```python
from build123d import *

# Parameters (mm, degrees)
SKETCH_1_W          = 37
SKETCH_1_H          = 30
SKETCH_1_R          = 1.5
EXTRUDE_1_DEPTH     = 10
SKETCH_2_R          = 1.5
CUT_EXTRUDE_1_DEPTH = 6
SKETCH_3_W          = 30
SKETCH_3_H          = 8
CUT_EXTRUDE_2_DEPTH = 3
SKETCH_4_R          = 1
CUT_EXTRUDE_3_DEPTH = 7


with BuildPart() as part:
    # Эскиз1 → Бобышка-Вытянуть1 (new body)
    with BuildSketch(Plane(origin=(0, 0, 0), x_dir=(1, 0, 0), z_dir=(0, 1, 0))):
        with Locations((18.5, 15)):
            Rectangle(SKETCH_1_W, SKETCH_1_H)
        with Locations(Location((26.949747468, 19.949747468, 0), (0, 0, 270))):
            Circle(SKETCH_1_R, mode=Mode.SUBTRACT)
        with Locations(Location((17.050252532, 19.949747468, 0), (0, 0, 270))):
            Circle(SKETCH_1_R, mode=Mode.SUBTRACT)
        with Locations(Location((26.949747468, 10.050252532, 0), (0, 0, 270))):
            Circle(SKETCH_1_R, mode=Mode.SUBTRACT)
        with Locations(Location((17.050252532, 10.050252532, 0), (0, 0, 270))):
            Circle(SKETCH_1_R, mode=Mode.SUBTRACT)
    extrude(amount=EXTRUDE_1_DEPTH)

    # Эскиз2 → Вырез-Вытянуть1 (cut)
    with BuildSketch(Plane(origin=(37, 0, 0), x_dir=(0, 0, -1), z_dir=(1, 0, 0))):
        with Locations((8, 5)):
            Circle(SKETCH_2_R)
        with Locations((22, 5)):
            Circle(SKETCH_2_R)
    extrude(amount=-CUT_EXTRUDE_1_DEPTH, mode=Mode.SUBTRACT)

    # Эскиз3 → Вырез-Вытянуть2 (cut)
    with BuildSketch(Plane.ZY):
        with Locations((-15, 6)):
            Rectangle(SKETCH_3_W, SKETCH_3_H)
    extrude(amount=-CUT_EXTRUDE_2_DEPTH, mode=Mode.SUBTRACT)

    # Эскиз4 → Вырез-Вытянуть3 (cut)
    with BuildSketch(Plane.ZY):
        with Locations((-20, 5.4)):
            Circle(SKETCH_4_R)
        with Locations((-10, 5.4)):
            Circle(SKETCH_4_R)
    extrude(amount=-CUT_EXTRUDE_3_DEPTH, mode=Mode.SUBTRACT)


solid = part.part
```
Could you check a few things on this model? Use its own coordinates, in mm. A direction names the side the tool comes from. Give positions to 0.01 mm unless a question says otherwise; leave off trailing zeros. Order: outer loops, then holes, each group sorted by start corner. A loop starts at its lowest first (then second) coordinate and runs counter-clockwise, first axis right, second up.
Q1. Suppose I cut it at B-B, the plane y = 5. Write out the boundary of the cut face in (x, z), and give its area (3 significant figures).
Q2. For faces 4 (the cylindrical face through (4.972, 4.424, -10.217)), 5 (the flat face through (3, 6, -15)), 6 (the flat face through (31, 5, -8)), which set-ups out of +Z, -Z, +X, -X, +Y, -Y let a thin tool reach every point of the face, with its end or its side?
Q3. Suppose I cut it at D-D, the plane x = 16.5. Write out the boundary of the cut face in (y, z), and give its area (3 significant figures).
Q4. If I drill on line 1 along Z through (x, y) = (17, 8); line 2 along X through (y, z) = (0.75, -20.5); line 3 along Z through (x, y) = (18, 3), over which ranges is the centre line in solid material (lowest first)?
Q5. I'm going to push flat-ended pins straight in: P1, Ø1.5, axis at y = 4.5, z = -8.5, coming from the +X side; P2, Ø3.5, axis at x = 1, z = -14, coming from the +Y side; P3, Ø4, axis at y = 7.5, z = -21.5, coming from the -X side. Where does each tip first touch, or does it pass through?
Q6. We'd pull the mould along Y, two halves only. Please class faces 1 (the flat face through (31, 5, -22)), 2 (the flat face through (1, 2, -15)), 3 (the flat face through (18, 5, 0)): +Y half, -Y half, draft (parallel to the pull), parting line (faces both ways), or undercut.
Q7. Suppose I cut it at A-A, the plane x = 3.5. Write out the boundary of the cut face in (y, z).
Q8. Suppose I cut it at C-C, the plane z = -8. Write out the boundary of the cut face in (x, y).
Solution:
1. outline: (3, -30) - (37, -30) - (37, -23.5) - (31, -23.5) - (31, -20.5) - (37, -20.5) - (37, -9.5) - (31, -9.5) - (31, -6.5) - (37, -6.5) - (37, 0) - (3, 0) - (3, -9.08) - (7, -9.08) - (7, -10.92) - (3, -10.92) - (3, -19.08) - (7, -19.08) - (7, -20.92) - (3, -20.92) - close; hole circle Ø3 at (17.05, -19.95); hole circle Ø3 at (17.05, -10.05); hole circle Ø3 at (26.95, -19.95); hole circle Ø3 at (26.95, -10.05)
1. area: 941 mm2
2. face 4: -X
2. face 5: +Z, -Z, -X, +Y
2. face 6: +X
3. outline: (0, -30) - (10, -30) - (10, -21.35) - (0, -21.35) - close; (0, -18.55) - (10, -18.55) - (10, -11.45) - (0, -11.45) - close; (0, -8.65) - (10, -8.65) - (10, 0) - (0, 0) - close
3. area: 244 mm2
4. line 1: z = -30 to -21.45, -18.45 to -11.55, -8.55 to 0
4. line 2: x = 0 to 15.65, 18.45 to 25.55, 28.35 to 37
4. line 3: z = -30 to -21.11, -18.79 to -11.21, -8.89 to 0
5. P1: stops at x = 31
5. P2: stops at y = 2
5. P3: stops at x = 3
6. face 1: undercut
6. face 2: +Y half
6. face 3: draft
7. outline: (0, -30) - (10, -30) - (10, 0) - (0, 0) - close; hole circle Ø2 at (5.4, -20); hole circle Ø2 at (5.4, -10)
8. outline: (0, 0) - (37, 0) - (37, 3.5) - (31, 3.5) - (31, 6.5) - (37, 6.5) - (37, 10) - (3, 10) - (3, 2) - (0, 2) - close
